Source: CAD feature listing. Evaluate the final solid. Frame: model axes, mm. Face numbers are marked on the shaded views. A direction names the side the tool comes from. Round coordinates to 2 decimals unless told otherwise and drop trailing zeros. Order: outer loops, then holes, each group sorted by start corner. A loop starts at its lowest first (then second) coordinate and runs counter-clockwise, first axis right, second up. Notation, with made-up numbers: (-22.5, 87.25) -> (25.5, 87.25) arc R36 cw to (25.5, 124.25) -> close; hole circle Ø6 at (44.5, -5). An arc over 180 degrees is marked (long way). Answer as CSV lines item,"result". Start each with the question number.
(1) Section query C-C (z = 12.75). Output: boundary loops of the cut face in (x, y).
(2) Section query A-A (y = 0). Output: boundary loops of the cut face in (x, z), plus the area to 3 significant figures.
(3) Contact query for a flat-ended pin moving along its axis: P1, Ø3, axis at x = -6.5, y = 4, coming from the +Z side. Output: stop coordinate, or through.
(4) Section query B-B (x = 0). Output: boundary loops of the cut face in (y, z), plus the area to 3 significant figures.
(5) Line query: line 1 along Z through (x, y) = (-4.5, -1); line 2 along X through (y, z) = (1, 13.5). Output: solid intervals per line, ascending. Write a range as from..to.
(6) Set-up query: the marked faces 1 and 2. Return all of +Z, -Z, +X, -X, +Y, -Y with unobstructed straight access to the full face (end or side cutting, diameter ignored); none if empty.
(7) Section query D-D (y = 5.5). Output: boundary loops of the cut face in (x, z).
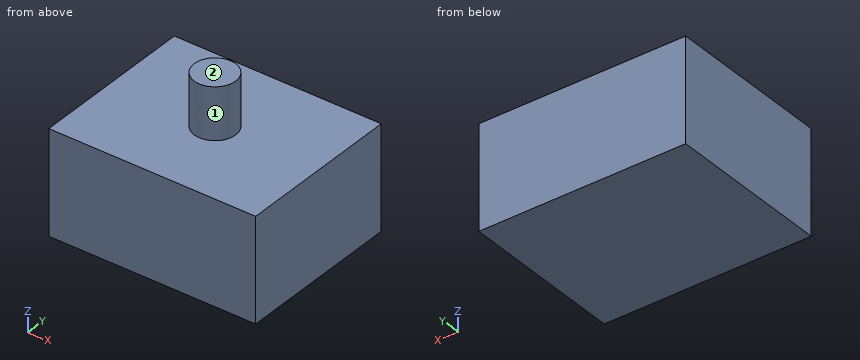
```python
from build123d import *

# Parameters (mm, degrees)
SKETCH1_W           = 20
SKETCH1_H           = 16
SKETCH1_R           = 2
BOSS_EXTRUDE1_DEPTH = 10
SKETCH1_3_R         = 2
BOSS_EXTRUDE2_DEPTH = 15


with BuildPart() as part:
    # Sketch1 → Boss-Extrude1 (new body)
    with BuildSketch(Plane.XY):
        Rectangle(SKETCH1_W, SKETCH1_H)
        Circle(SKETCH1_R, mode=Mode.SUBTRACT)
    extrude(amount=BOSS_EXTRUDE1_DEPTH)

    # Sketch1_3 → Boss-Extrude2 (add)
    with BuildSketch(Plane.XY):
        Circle(SKETCH1_3_R)
    extrude(amount=BOSS_EXTRUDE2_DEPTH)


solid = part.part
```
Answer block:
1,outline,"circle Ø4 at (0, 0)"
2,outline,"(-10, 0) -> (10, 0) -> (10, 10) -> (2, 10) -> (2, 15) -> (-2, 15) -> (-2, 10) -> (-10, 10) -> close"
2,area,"220 mm2"
3,P1,"z = 10"
4,outline,"(-8, 0) -> (8, 0) -> (8, 10) -> (2, 10) -> (2, 15) -> (-2, 15) -> (-2, 10) -> (-8, 10) -> close"
4,area,"180 mm2"
5,line 1,"0..10"
5,line 2,"-1.73..1.73"
6,face 1,"+Z"
6,face 2,"+Z, +X, -X, +Y, -Y"
7,outline,"(-10, 0) -> (10, 0) -> (10, 10) -> (-10, 10) -> close"
